Verification items for this drawing (mm, ordinates from the low corner). Round coordinates to 2 decimals unless told otherwise and drop trailing zeros. Loops run counter-clockwise (first coordinate to the right, second up) from the corner with the lowest first, then second, coordinate; pieces in that order, holes last. Notation, with made-up numbers: M 69.5,-22 L 127.5,-22 A9 ccw 127.5,-18 Z; hole C 13,-24 d1. An arc over 180 degrees is marked long. Answer as CSV lines item,"result".
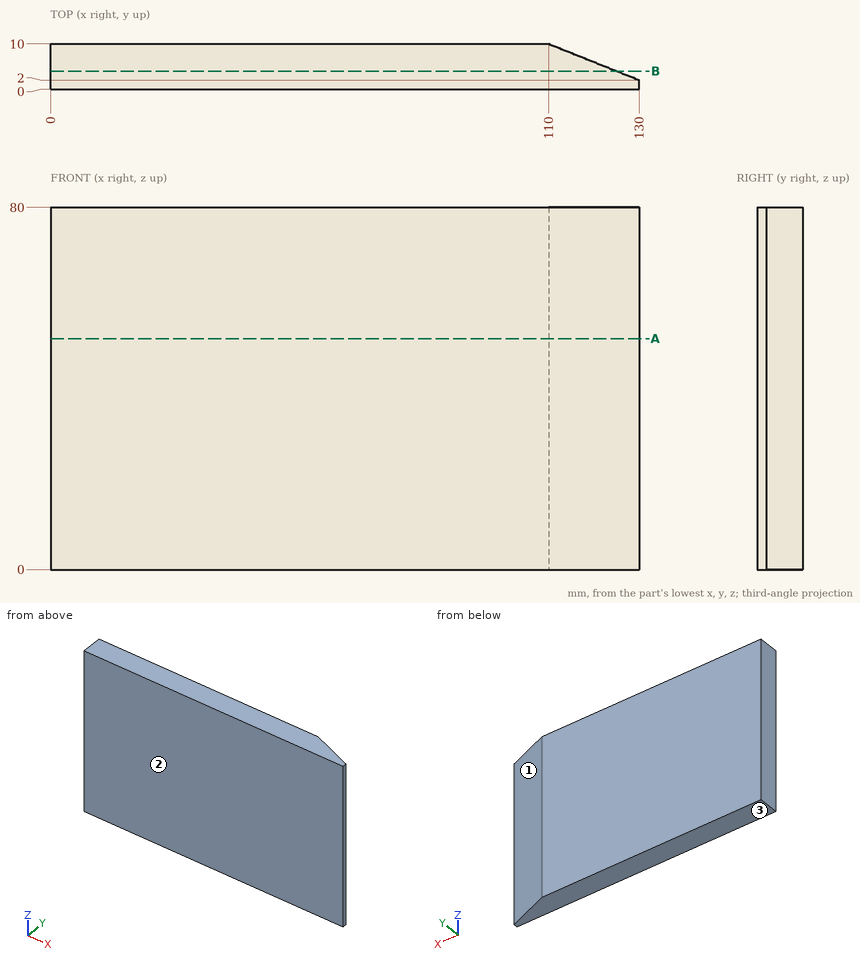
1) Section check A-A (z = 51). Record the cut outline in (x, y), plus the area to 3 significant figures.
Here are the results:
outline,"M 0,0 L 130,0 L 130,2 L 110,10 L 0,10 Z"
area,"1,220 mm^2"
2) Draft check along Y on the marked faces 1, 2 and 3. Enter one of: +Y half, -Y half, draft (parallel to the pull), parting line (faces both ways), or undercut.
Here are the results:
face 1,"+Y half"
face 2,"-Y half"
face 3,"draft"
3) Section check B-B (y = 4). Record the cut outline in (x, z).
Here are the results:
outline,"M 0,0 L 125,0 L 125,80 L 0,80 Z"
